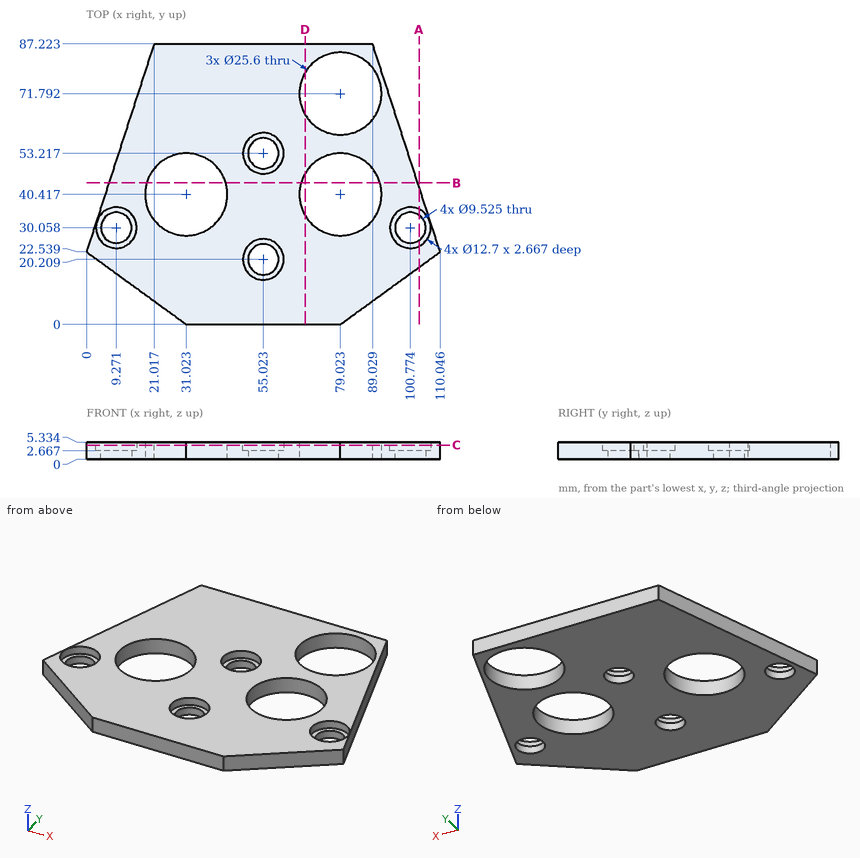
Here's the drawing with two shaded views (mm, measured from the low corner). I have some questions. Give positions to 0.01 mm unless a question says otherwise; leave off trailing zeros. Loops run counter-clockwise (first coordinate to the right, second up) from the corner with the lowest first, then second, coordinate; pieces in that order, holes last. Notation, with made-up numbers: (77, -12.75) -> (99, -12.75) arc R3 cw to (99, -8.75) -> close; hole circle Ø3 at (60.25, 33). An arc over 180 degrees is marked (long way). One line per item, written item: value.
Q1. Suppose I cut it at C-C on z = 4.5. State how many separate pieces and enclosed holes the cut face has, then the cut area to 3 significant figures.
Answers follow:
separate pieces: 1
enclosed holes: 7
area: 5,490 mm^2
Q2. Suppose I cut it at B-B on y = 44. Please give me the cut outline in (x, z) (1 decimal).
Answers follow:
outline: (7, 0) -> (18.7, 0) -> (18.7, 5.3) -> (7, 5.3) -> close; (43.3, 0) -> (66.7, 0) -> (66.7, 5.3) -> (43.3, 5.3) -> close; (91.3, 0) -> (103.1, 0) -> (103.1, 5.3) -> (91.3, 5.3) -> close
Q3. I'm going to push flat-ended pins straight in: pin 1 Ø14.5 at (x, y) = (100.77, 30.06) entering from -Z; pin 2 Ø6.5 at (x, y) = (56, 56) entering from +Z; pin 3 Ø1.5 at (y, z) = (9, 3) entering from +X. Where does each tip first touch, or does it pass through?
Answers follow:
pin 1: z = 0
pin 2: z = 2.67
pin 3: x = 92.44
Q4. If I drill on line 1 along Y through (x, z) = (73, 3.9) (1 decimal); line 2 along X through (y, z) = (50.5, 4.2) (1 decimal); line 3 along Y through (x, z) = (77, 2.65), over which ranges is the centre line in solid material (lowest first)?
Answers follow:
line 1: 0 to 29.1, 51.7 to 60.5, 83.1 to 87.2
line 2: 9.1 to 23.1, 38.9 to 49.3, 60.8 to 71.1, 86.9 to 101
line 3: 0 to 27.78, 53.06 to 59.15, 84.43 to 87.22
Q5. Suppose I cut it at D-D on x = 68. Please give me the cut outline in (y, z) (1 decimal).
Answers follow:
outline: (0, 0) -> (33.9, 0) -> (33.9, 5.3) -> (0, 5.3) -> close; (46.9, 0) -> (65.3, 0) -> (65.3, 5.3) -> (46.9, 5.3) -> close; (78.3, 0) -> (87.2, 0) -> (87.2, 5.3) -> (78.3, 5.3) -> close
Q6. Suppose I cut it at A-A on x = 103.5. Please give me the cut outline in (y, z) (1 decimal).
Answers follow:
outline: (17.8, 0) -> (26.2, 0) -> (26.2, 2.7) -> (24.3, 2.7) -> (24.3, 5.3) -> (17.8, 5.3) -> close; (34, 0) -> (42.7, 0) -> (42.7, 5.3) -> (35.8, 5.3) -> (35.8, 2.7) -> (34, 2.7) -> close
